Here's how the part is built. I have some questions about the finished solid (model axes, mm). Face numbers are marked on the shaded views. Round coordinates to 2 decimals unless told otherwise and drop trailing zeros. Write each loop counter-clockwise with the first axis right and the second up, starting at its lowest first coordinate (ties: lowest second). Pieces come first, ordered by that corner, then holes. Notation, with made-up numbers: (43.5, 49) - (51.5, 49) arc R25 ccw to (51.5, 66) - close; hole circle Ø11 at (-4.75, 47). An arc over 180 degrees is marked (long way). Write item = value, one per line. Start each with the question number.
Item 1: Thinking about a two-plate mould opening in X: for the marked faces 1 and 2, which applies, pulls with the +X half, pulls with the -X half, needs draft (parallel to the pull), parting line crosses it, or undercut?
Item 2: If we section it at A-A (y = 12.7): Give the number of separate pieces and of enclosed holes in the cut face, and give its area (3 significant figures).
Item 3: If we section it at C-C (x = 13.17): Please give me the cut outline in (y, z) (1 decimal).
Item 4: If we section it at D-D (y = 16): Please give me the cut outline in (x, z) (3 decimals), and give its area (3 significant figures).
Item 5: If I drill on line 1 along Y through (x, z) = (13.17, 1); line 2 along X through (y, z) = (8.75, -1.25); line 3 along X through (y, z) = (11.75, 0.75), over which ranges is the centre line in solid material (lowest first)? Write a range as [from, to].
```python
from build123d import *

# Parameters (mm, degrees)
SKETCH1_W             = 87.3
SKETCH1_H             = 25.4
SKETCH1_R             = 4.7625
BOSS_EXTRUDE1_DEPTH   = 3.175
F_6_CLEARANCE_HOLE1_D = 3.6576


with BuildPart() as part:
    # Sketch1 → Boss-Extrude1 (new, symmetric)
    with BuildSketch(Plane.XY):
        with Locations((0, 12.7)):
            Rectangle(SKETCH1_W, SKETCH1_H)
        with Locations((13.17, 12.7)):
            Circle(SKETCH1_R, mode=Mode.SUBTRACT)
    extrude(amount=BOSS_EXTRUDE1_DEPTH, both=True)

    # #6 Clearance Hole1 (through all)
    with Locations(Plane.XY.offset(3.175)):
        with Locations((-38.8875, 12.7), (38.8875, 12.7)):
            Hole(F_6_CLEARANCE_HOLE1_D / 2)


solid = part.part
```
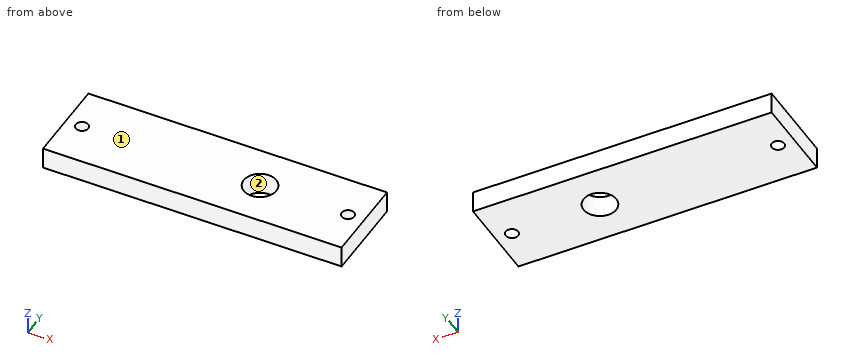
Reply:
q1.face_1 = needs draft
q1.face_2 = undercut
q2.separate_pieces = 4
q2.enclosed_holes = 0
q2.area = 447 mm2
q3.outline = (0, -3.2) - (7.9, -3.2) - (7.9, 3.2) - (0, 3.2) - close; (17.5, -3.2) - (25.4, -3.2) - (25.4, 3.2) - (17.5, 3.2) - close
q4.outline = (-43.65, -3.175) - (9.736, -3.175) - (9.736, 3.175) - (-43.65, 3.175) - close; (16.604, -3.175) - (43.65, -3.175) - (43.65, 3.175) - (16.604, 3.175) - close
q4.area = 511 mm2
q5.line_1 = [0, 7.94], [17.46, 25.4]
q5.line_2 = [-43.65, 10.51], [15.83, 43.65]
q5.line_3 = [-43.65, -40.45], [-37.32, 8.5], [17.84, 37.32], [40.45, 43.65]
